Verification items for the finished model (mm, model axes). Round coordinates to 2 decimals unless told otherwise and drop trailing zeros.
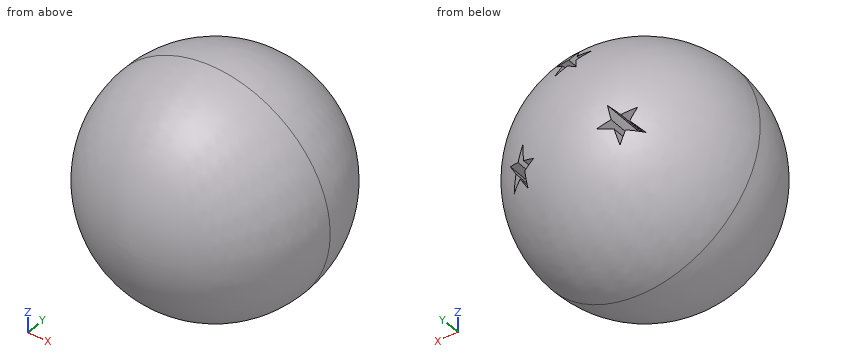
```python
from build123d import *

# Parameters (mm, degrees)
F3_DEPTH = 50.8


with BuildPart() as f1:
    # F0 (on Top) → F1 (revolve)
    with BuildSketch(Plane.XY):
        with BuildLine():
            Line((0, 38.1), (0, 0))
            Line((0, 0), (38.1, 0))
            ThreePointArc((38.1, 0), (26.940768, 26.940768), (0, 38.1))
        make_face()
    revolve(axis=Axis((0, 19.05, 0), (0, 1, 0)))

    # F2 (on face) → F3 (cut)
    with BuildSketch(Plane.XZ):
        Polygon((0, 25.153092), (0, 16.718826), (3.587308, 14.112495), (2.217078, 18.329628), (5.804386, 20.935959), (1.37023, 20.935959), align=None)
        Polygon((-3.587308, 14.112495), (0, 16.718826), (0, 25.153092), (-1.37023, 20.935959), (-5.804386, 20.935959), (-2.217078, 18.329628), align=None)
        Polygon((-18.816187, -9.281326), (-21.783217, -12.576546), (-17.445958, -11.654633), (-15.22888, -15.494725), (-14.765384, -11.08486), (-10.428125, -10.162947), (-14.478928, -8.359413), (-14.015433, -3.949548), (-16.982462, -7.244768), (-21.033265, -5.441234), align=None)
        Polygon((17.445958, -11.654633), (21.783217, -12.576546), (18.816187, -9.281326), (21.033265, -5.441234), (16.982462, -7.244768), (14.015433, -3.949548), (14.478928, -8.359413), (10.428125, -10.162947), (14.765384, -11.08486), (15.22888, -15.494725), align=None)
    extrude(amount=-F3_DEPTH, mode=Mode.SUBTRACT)

    # F4 (on Top) → F5 (revolve)
    with BuildSketch(Plane.XY):
        with BuildLine():
            Line((38.1, 0), (0, 0))
            Line((0, 0), (0, -38.1))
            ThreePointArc((0, -38.1), (26.940768, -26.940768), (38.1, 0))
        make_face()
    revolve(axis=Axis((0, -19.05, 0), (0, -1, 0)))


solid = f1.part
```
1) Go/stop test with flat-tipped pins: pin 1 Ø10 at (y, z) = (-12.5, -16) entering from -X; pin 2 Ø2 at (x, y) = (-4.5, 21.5) entering from -Z; pin 3 Ø3.5 at (x, z) = (15, -8) entering from +Y. Record where each tip stops, or that it passes through.
2) Sectioned sample at A-A on y = 15.5. Count the separate pieces of the cut face and the enclosed holes in it, then the cut area to 3 significant figures.
3) Scan lines: probe 1 along Z at (x, y) = (-13.5, 12); probe 2 along X at (y, z) = (-1, -6.5); probe 3 along X at (y, z) = (-2, 10). Record each from-to range of solid material in increasing order.
Returned:
1. pin 1: stops at x = -34.89
1. pin 2: stops at z = -31.81
1. pin 3: stops at y = 34.91
2. separate pieces: 1
2. enclosed holes: 3
2. area: 3,680 mm2
3. probe 1: z = -33.55 to -10.82, -8.8 to 33.55
3. probe 2: x = -37.53 to 37.53
3. probe 3: x = -36.71 to 36.71
